Input: dimensioned drawing with shaded views. Units: mm. Origin: part minimum x, y, z. A direction names the side the tool comes from. Round coordinates to 2 decimals unless told otherwise and drop trailing zeros. Loops run counter-clockwise (first coordinate to the right, second up) from the corner with the lowest first, then second, coordinate; pieces in that order, holes last. Notation, with made-up numbers: M -28.5,11.5 L -24.5,11.5 A25 cw -24.5,28.5 Z; hole C 17.25,-1 d6. An arc over 180 degrees is marked long. Answer as CSV lines item,"result". Start each with the question number.
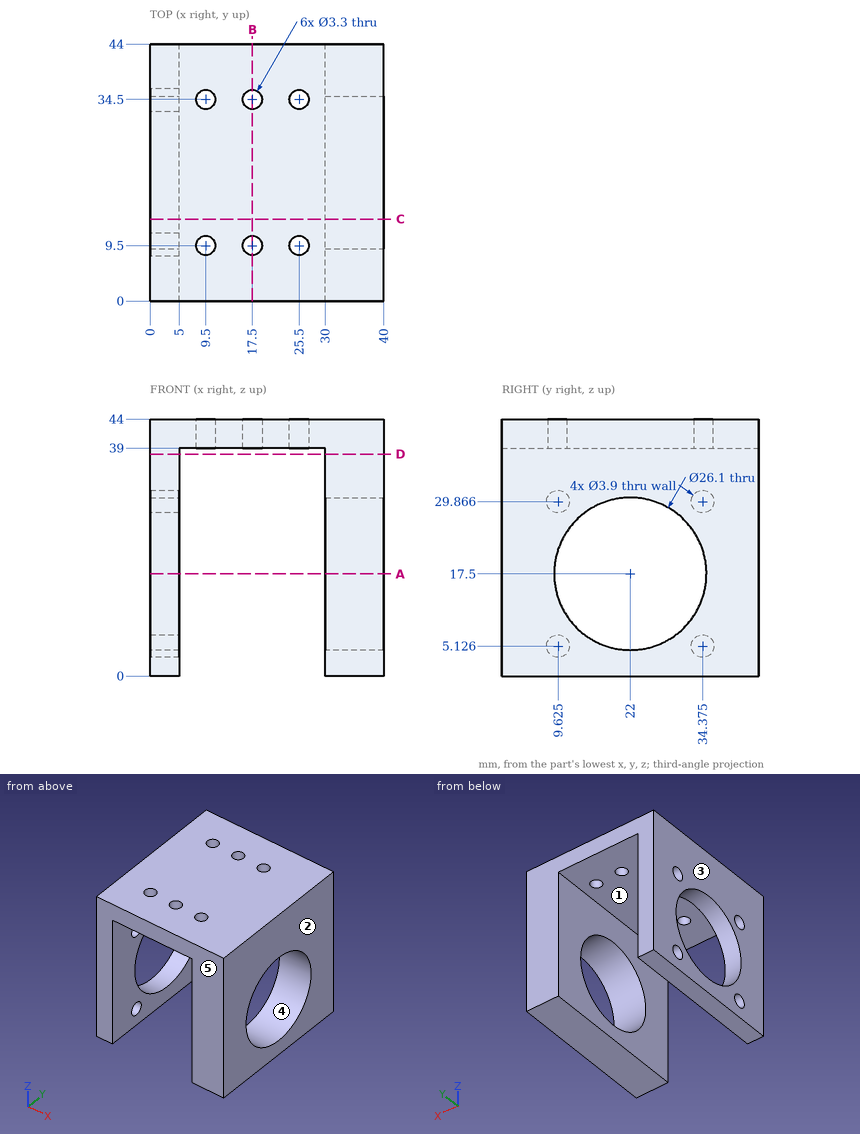
1) Mould query, pull axis Y, two halves, no side actions, for the marked faces 3, 4 and 5. Classes: pulls with the +Y half, pulls with the -Y half, needs draft (parallel to the pull), parting line crosses it, or undercut.
2) Contact query for flat-ended pins moving along their axis: pin 1 Ø3.5 at (y, z) = (34.38, 29.87) entering from -X; pin 2 Ø5 at (x, y) = (16.5, 10) entering from +Z; pin 3 Ø4 at (x, y) = (9.5, 9.5) entering from -Z. Output: stop coordinate, or through.
3) Section B-B, the plane x = 17.5. Return loops of the section in (y, z).
4) Section D-D, the plane z = 38. Return loops of the section in (x, y).
5) Section C-C, the plane y = 14. Return loops of the section in (x, z), and give its area (3 significant figures).
6) Section A-A, the plane z = 17.5. Return loops of the section in (x, y).
7) Ray query, line 1 along X through (y, z) = (6, 38); line 2 along Y through (x, z) = (25.5, 42.45); line 3 along Z through (x, y) = (13.5, 30). Return the intervals inside material, ascending.
8) Access query for the marked faces 1 and 2. Directions: +Z, -Z, +X, -X, +Y, -Y. A direction counts if a zero-diameter tool reaches every point of the face in a straight line with its end or side. Return the directions, or none.
Findings below:
1,face 3,"needs draft"
1,face 4,"undercut"
1,face 5,"pulls with the -Y half"
2,pin 1,"x = 30"
2,pin 2,"z = 44"
2,pin 3,"z = 39"
3,outline,"M 0,39 L 7.85,39 L 7.85,44 L 0,44 Z; M 11.15,39 L 32.85,39 L 32.85,44 L 11.15,44 Z; M 36.15,39 L 44,39 L 44,44 L 36.15,44 Z"
4,outline,"M 0,0 L 5,0 L 5,44 L 0,44 Z; M 30,0 L 40,0 L 40,44 L 30,44 Z"
5,outline,"M 0,0 L 5,0 L 5,7.19 L 0,7.19 Z; M 0,27.81 L 5,27.81 L 5,39 L 30,39 L 30,27.81 L 40,27.81 L 40,44 L 0,44 Z; M 30,0 L 40,0 L 40,7.19 L 30,7.19 Z"
5,area,"476 mm²"
6,outline,"M 0,0 L 5,0 L 5,8.95 L 0,8.95 Z; M 0,35.05 L 5,35.05 L 5,44 L 0,44 Z; M 30,0 L 40,0 L 40,8.95 L 30,8.95 Z; M 30,35.05 L 40,35.05 L 40,44 L 30,44 Z"
7,line 1,"0 to 5, 30 to 40"
7,line 2,"0 to 7.85, 11.15 to 32.85, 36.15 to 44"
7,line 3,"39 to 44"
8,face 1,"-Z, +Y, -Y"
8,face 2,"+Z, -Z, +X, +Y, -Y"
